Can you work these out from the model? Positions are in its coordinate system, mm. A direction names the side the tool comes from. Give positions to 0.01 mm unless a question says otherwise; leave off trailing zeros. Order: outer loops, then holes, each group sorted by start corner. A loop starts at its lowest first (then second) coordinate and runs counter-clockwise, first axis right, second up. Notation, with made-up numbers: (-1.5, 29) - (53.5, 29) arc R13 cw to (53.5, 35) - close; hole circle Ø4 at (83.25, -31.75). An arc over 180 degrees is marked (long way). Use one line per item in the form item = value. Start each with the question number.
1) Please list where these lines run through material, in increasing order: probe 1 along Y at (x, z) = (-14.5, 1.9); probe 2 along X at (y, z) = (-4, 1.3); probe 3 along Y at (x, z) = (-0.5, 2.2).
2) We'd pull the mould along Y, two halves only. Please class faces 1 (the flat face through (-25, 17, 2)), 2 (the flat face through (-15, 30, 2)), 3 (the flat face through (-30, 0, 2)): released by +Y, released by -Y, zero draft, split by the parting line, or undercut.
3) Suppose I cut it at A-A, the plane y = -5. Write out the boundary of the cut face in (x, z), and give its area (3 significant figures).
4) Suppose I cut it at D-D, the plane y = 21. Write out the boundary of the cut face in (x, z).
5) Suppose I cut it at C-C, the plane z = 2.8. State how many separate pieces and enclosed holes the cut face has, and give its area (3 significant figures).
6) Which directions (+Z, -Z, +X, -X, +Y, -Y) give clear straight access to the entire face, cutting with the end or side of a thin tool? Please do faces 4 (the flat face through (-25, -17, 2)), 5 (the flat face through (-30, 26, 2)).
7) Suppose I cut it at B-B, the plane x = 8.5. Write out the boundary of the cut face in (y, z), and give its area (3 significant figures).
8) For pin 1 (2 mm diameter, centred on y = 15.5, z = 2.5, fed in from +X); pin 2 (8 mm diameter, centred on x = -14.5, y = 14.5, fed in from +Z); pin 3 (3 mm diameter, centred on x = -14.5, y = -14.5, fed in from -Z); pin 4 (1.5 mm diameter, centred on y = 18, z = 3.5, fed in from -X), each with a flat end and sliding along its axis, tell me the tip position at first contact or that it passes through.
```python
from build123d import *

# Parameters (mm, degrees)
SKETCH1_R           = 16
SKETCH1_R_2         = 2.5
BOSS_EXTRUDE1_DEPTH = 5
FILLET1_R           = 30


with BuildPart() as part:
    # Sketch1 → Boss-Extrude1 (new body)
    with BuildSketch(Plane(origin=(0, 0, 0), x_dir=(0, 1, 0), z_dir=(0, 0, 1))):
        Polygon((-30, -30), (30, -30), (30, 30), (22, 30), (22, 25), (12, 25), (12, 30), (-12, 30), (-12, 25), (-22, 25), (-22, 30), (-30, 30), align=None)
        with Locations(Location((0, 0, 0), (0, 0, 270))):
            Circle(SKETCH1_R, mode=Mode.SUBTRACT)
        with Locations(Location((14.495689014, 14.495689014, 0), (0, 0, 270))):
            Circle(SKETCH1_R_2, mode=Mode.SUBTRACT)
        with Locations(Location((14.495689014, -14.495689014, 0), (0, 0, 270))):
            Circle(SKETCH1_R_2, mode=Mode.SUBTRACT)
        with Locations(Location((-14.495689014, -14.495689014, 0), (0, 0, 270))):
            Circle(SKETCH1_R_2, mode=Mode.SUBTRACT)
        with Locations(Location((-14.495689014, 14.495689014, 0), (0, 0, 270))):
            Circle(SKETCH1_R_2, mode=Mode.SUBTRACT)
    extrude(amount=BOSS_EXTRUDE1_DEPTH)

    # Fillet1
    fillet1_edges = [part.edges().sort_by_distance(p)[0] for p in [
        (30, 30, 2.5),
        (30, -30, 2.5),
    ]]
    fillet(fillet1_edges, radius=FILLET1_R - 0.0001)  # a hair under: the kernel refuses the full size


solid = part.part
```
Result sheet:
q1.probe_1 = -30 to -17, -12 to -6.76, 6.76 to 12, 17 to 30
q1.probe_2 = -30 to -15.49, 15.49 to 29.73
q1.probe_3 = -30 to -15.99, 15.99 to 30
q2.face_1 = undercut
q2.face_2 = released by +Y
q2.face_3 = zero draft
q3.outline = (-30, 0) - (-15.2, 0) - (-15.2, 5) - (-30, 5) - close; (15.2, 0) - (29.58, 0) - (29.58, 5) - (15.2, 5) - close
q3.area = 146 mm²
q4.outline = (-25, 0) - (21.42, 0) - (21.42, 5) - (-25, 5) - close
q5.separate_pieces = 1
q5.enclosed_holes = 5
q5.area = 2,230 mm²
q6.face_4 = +Z, -Z, -X
q6.face_5 = +Z, -Z, -X, +Y, -Y
q7.outline = (-28.77, 0) - (-13.56, 0) - (-13.56, 5) - (-28.77, 5) - close; (13.56, 0) - (28.77, 0) - (28.77, 5) - (13.56, 5) - close
q7.area = 152 mm²
q8.pin_1 = 26.26
q8.pin_2 = 5
q8.pin_3 = through
q8.pin_4 = -25
